The listing builds one solid part. Answer for the finished solid, in the listing's coordinates (mm). Face numbers are marked on the shaded views. A direction names the side the tool comes from. Give positions to 0.01 mm unless a question says otherwise; leave off trailing zeros. Write each loop counter-clockwise with the first axis right and the second up, starting at its lowest first coordinate (ties: lowest second). Pieces come first, ordered by that corner, then holes. Notation, with made-up numbers: (-18.5, -18) - (6.5, -18) arc R17 cw to (6.5, -8) - close; hole circle Ø7 at (12, 60). An arc over 180 degrees is marked (long way). Return JSON: item names as keys, results as strings.
from build123d import *

# Parameters (mm, degrees)
SKETCH1_W           = 20
SKETCH1_H           = 20
BOSS_EXTRUDE1_DEPTH = 3
FILLET1_R           = 1
SKETCH2_R           = 2.5
BOSS_EXTRUDE2_DEPTH = 5


with BuildPart() as part:
    # Sketch1 → Boss-Extrude1 (new body)
    with BuildSketch(Plane(origin=(0, 0, 0), x_dir=(1, 0, 0), z_dir=(0, 1, 0))):
        Rectangle(SKETCH1_W, SKETCH1_H)
    extrude(amount=BOSS_EXTRUDE1_DEPTH)

    # Fillet1
    fillet1_edges = [part.edges().sort_by_distance(p)[0] for p in [
        (-10, 3, 0),
        (0, 3, 10),
        (10, 3, 0),
        (0, 3, -10),
    ]]
    fillet(fillet1_edges, radius=FILLET1_R)

    # Sketch2 → Boss-Extrude2 (add)
    with BuildSketch(Plane.XZ):
        Circle(SKETCH2_R)
    extrude(amount=BOSS_EXTRUDE2_DEPTH)


solid = part.part
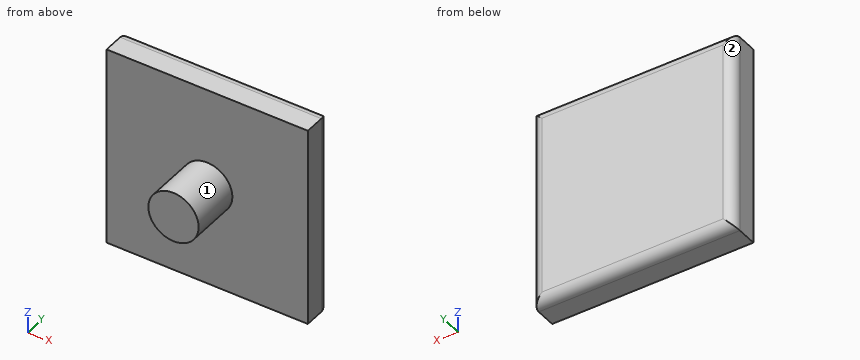
Item 1: Consider L1, parallel to Y at x = -4.5, z = -8.25; L2, parallel to Z at x = -1.5, y = -2.5; L3, parallel to Z at x = 1.75, y = -0.25. Determine where each line is inside the solid, lowest interval first.
Answer below:
{"L1": "y = 0 to 3", "L2": "z = -2 to 2", "L3": "z = -1.79 to 1.79"}
Item 2: A cutting plane is placed at B-B on z = 0. Determine the outline of the cut face in (x, y), then the cut area to 3 significant figures.
Answer below:
{"outline": "(-10, 0) - (-2.5, 0) - (-2.5, -5) - (2.5, -5) - (2.5, 0) - (10, 0) - (10, 2) arc R1 ccw to (9, 3) - (-9, 3) arc R1 ccw to (-10, 2) - close", "area": "84.6 mm²"}
Item 3: A flat-ended cylindrical pin translates along its axis: P1, Ø1, axis at x = 6, y = -2, coming from the +Z side. Find the tip coordinate at first contact, or state that the pin passes through.
Answer below:
{"P1": "passes through"}
Item 4: A cutting plane is placed at C-C on y = -3.25. Determine the outline of the cut face in (x, z), then the cut area to 3 significant figures.
Answer below:
{"outline": "circle Ø5 at (0, 0)", "area": "19.6 mm²"}
Item 5: A cutting plane is placed at D-D on z = 5.5. Determine the outline of the cut face in (x, y), then the cut area to 3 significant figures.
Answer below:
{"outline": "(-10, 0) - (10, 0) - (10, 2) arc R1 ccw to (9, 3) - (-9, 3) arc R1 ccw to (-10, 2) - close", "area": "59.6 mm²"}
Item 6: For the marked faces 1 and 2, determine the directions among +Z, -Z, +X, -X, +Y, -Y from which every point of the face is accessible in a straight line to the end or side of a thin tool.
Answer below:
{"face 1": "-Y", "face 2": "+Z, -Z, -X, +Y"}
Item 7: A cutting plane is placed at A-A on x = 0. Determine the outline of the cut face in (y, z), then the cut area to 3 significant figures.
Answer below:
{"outline": "(-5, -2.5) - (0, -2.5) - (0, -10) - (2, -10) arc R1 ccw to (3, -9) - (3, 9) arc R1 ccw to (2, 10) - (0, 10) - (0, 2.5) - (-5, 2.5) - close", "area": "84.6 mm²"}
